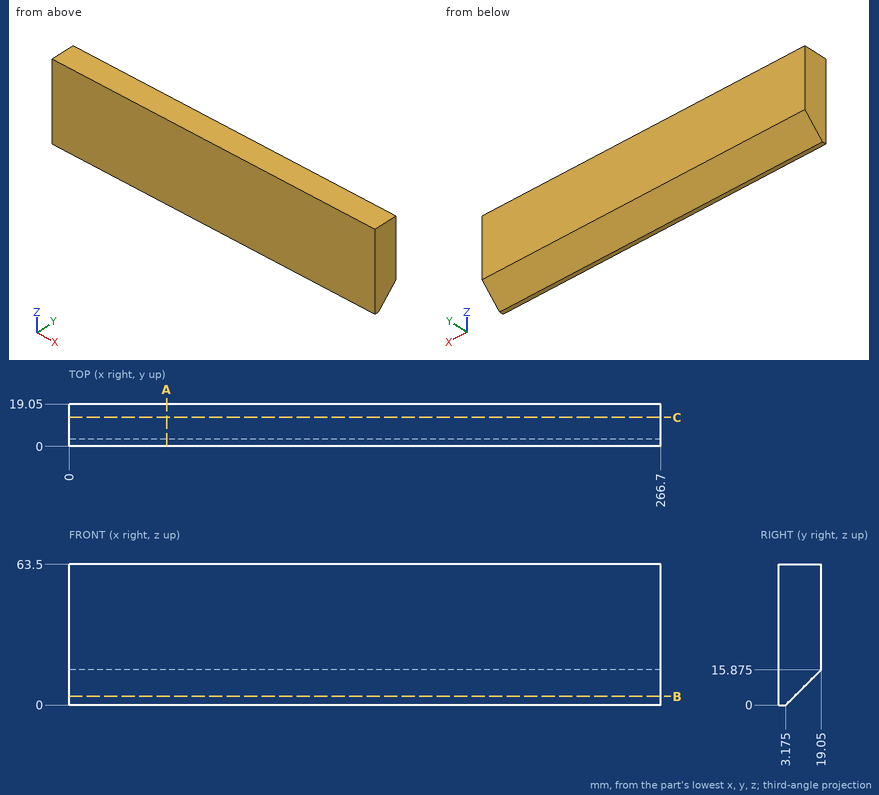
Geometry: see drawing. Coordinates: mm, zero at the bounding-box minimum. Give positions to 0.01 mm unless a question says otherwise; leave off trailing zeros. Order: outer loops, then holes, each group sorted by start corner. A loop starts at its lowest first (then second) coordinate and runs counter-clockwise, first axis right, second up. Notation, with made-up numbers: (61, -39.5) -> (108, -39.5) arc R16 ccw to (108, -11.5) -> close; hole circle Ø8 at (-16, -33.75). An arc over 180 degrees is marked (long way). Write each question's results on one line, items separated by ' | '. Start each with the question number.
1) First-contact query: pin 1 (8 mm diameter, centred on x = 104, z = 8.5, fed in from +Y) (3 decimals); pin 2 (3 mm diameter, centred on x = 124.5, y = 9.5, fed in from -Z) (3 decimals). Flat tips, straight axial feed; report the tip coordinate or a pass-through.
2) Section A-A (x = 44). Return loops of the section in (y, z) (3 decimals).
3) Section B-B (z = 4). Return loops of the section in (x, y) (3 decimals), then the cut area to 3 significant figures.
4) Line query: line 1 (Z direction, x = 121, y = 17.5) (3 decimals); line 2 (Z direction, x = 11.5, y = 4) (3 decimals); line 3 (Y direction, x = 148.5, z = 5.5) (3 decimals). Output: solid intervals per line, ascending. Write a range as from..to.
5) Section C-C (y = 13). Return loops of the section in (x, z) (3 decimals).
Calculated:
1) pin 1: y = 15.675 | pin 2: z = 4.825
2) outline: (0, 0) -> (3.175, 0) -> (19.05, 15.875) -> (19.05, 63.5) -> (0, 63.5) -> close
3) outline: (0, 0) -> (266.7, 0) -> (266.7, 7.175) -> (0, 7.175) -> close | area: 1,910 mm2
4) line 1: 14.325..63.5 | line 2: 0.825..63.5 | line 3: 0..8.675
5) outline: (0, 9.825) -> (266.7, 9.825) -> (266.7, 63.5) -> (0, 63.5) -> close
